Source: CAD feature listing. Evaluate the final solid. Frame: model axes, mm. A direction names the side the tool comes from. Round coordinates to 2 decimals unless told otherwise and drop trailing zeros. Write each loop counter-clockwise with the first axis right and the second up, starting at its lowest first coordinate (ties: lowest second). Pieces come first, ordered by that corner, then holes. Notation, with made-up numbers: (10.25, 33.25) -> (53.25, 33.25) arc R32 ccw to (53.25, 59.25) -> close; hole circle Ø10 at (9.25, -26.75). An arc over 180 degrees is marked (long way). Put each result on its own line as item: value.
Autodesk Inventor part; units mm, degrees
ref_plane "YZ Plane" through (0, 0, 0) normal (1, 0, 0) x (0, 1, 0)
ref_plane "XZ Plane" through (0, 0, 0) normal (0, 1, 0) x (-1, 0, 0)
ref_plane "XY Plane" through (0, 0, 0) normal (0, 0, 1) x (1, 0, 0)
sketch "Sketch1" plane through (0, 0, 0) normal (0, 0, 1) x (1, 0, 0)
  line L0 (-30, 0) -> (30, 0) construction
  line L1 (-30, -11) -> (30, -11)
  line L2 (30, 11) -> (-30, 11)
  arc A0 (-30, 11) -> (-30, -11) centre (-30, 0) ccw
  arc A1 (30, -11) -> (30, 11) centre (30, 0) ccw
  point P0 (0, 0)
  point P1 (0, 0)
  dimension "d0" = 22
  dimension "d1" = 60
extrude "Extrusion1" add sketch "Sketch1" along normal mid plane 92
sketch "Sketch2" plane through (0, 0, 46) normal (0, 0, 1) x (1, 0, 0)
  line L0 (19, 2.5) -> (31, 2.5)
  line L1 (31, 2.5) -> (31, -2.5)
  line L2 (31, -2.5) -> (19, -2.5)
  line L3 (19, -2.5) -> (19, 2.5)
  line L4 (19, 2.5) -> (31, -2.5) construction
  line L5 (31, 2.5) -> (19, -2.5) construction
  arc A0 (30, -11) -> (30, 11) centre (30, 0) ccw
  line L6 (30, 11) -> (-30, 11)
  arc A1 (-30, 11) -> (-30, -11) centre (-30, 0) ccw
  line L7 (-30, -11) -> (30, -11)
  line L8 (-29, 0) -> (-21, 0) construction
  line L9 (-29, -1.5) -> (-21, -1.5)
  line L10 (-21, 1.5) -> (-29, 1.5)
  arc A2 (-29, 1.5) -> (-29, -1.5) centre (-29, 0) ccw
  arc A3 (-21, -1.5) -> (-21, 1.5) centre (-21, 0) ccw
  point P0 (0, 0)
  point P1 (25, 0)
  point P2 (-25, 0)
  dimension "d4" = 5
  dimension "d5" = 12
  dimension "d6" = 25
  dimension "d13" = 3
  dimension "d14" = 8
  dimension "d15" = 25
extrude "Extrusion2" cut sketch "Sketch2" against normal blind 10 contours L0 L1 L2 L3 | A2 L10 A3 L9
sketch "Sketch3" plane through (-30, 11, 46) normal (0, 1, 0) x (1, 0, 0)
  circle A0 centre (30, 18.5011) radius 7.5
  point P0 (30, 46)
  dimension "d9" = 15
extrude "Extrusion3" cut sketch "Sketch3" against normal blind 1
fillet "Fillet1" radius 1 1 edges at (-7.5, 10, 27.4989)
properties part number "power-bank"
Q1. Material intervals for line 1 (X direction, y = 0.25, z = -34.5); line 2 (Y direction, x = -32.5, z = -18.5); line 3 (X direction, y = 8.5, z = 38.5), sorted ascending. Write a range as [from, to].
Ans:
line 1: x = [-41, 41]
line 2: y = [-10.71, 10.71]
line 3: x = [-36.98, 36.98]
Q2. Pin query (flat end, axial travel): pin 1 (6.5 mm diameter, centred on x = -0.5, z = 25, fed in from +Y); pin 2 (4 mm diameter, centred on x = 26, y = 0, fed in from +Z); pin 3 (6 mm diameter, centred on y = 6, z = 3, fed in from +X). Return the tip coordinate at first contact, or that it passes through.
Ans:
pin 1: stops at y = 10
pin 2: stops at z = 36
pin 3: stops at x = 40.58
Q3. Reachability of faces 1 (the flat face through (-1, 0, -46)), 2 (the flat face through (-25, -1.5, 41)) from +Z, -Z, +X, -X, +Y, -Y: full face, straight path, thin tool, end or side. Return the list, or none.
Ans:
face 1: -Z, +X, -X, +Y, -Y
face 2: +Z
Q4. Cut plane A-A on y = 0. Output: boundary loops of the cut face in (x, z), and give its area (3 significant figures).
Ans:
outline: (-41, -46) -> (41, -46) -> (41, 46) -> (31, 46) -> (31, 36) -> (19, 36) -> (19, 46) -> (-19.5, 46) -> (-19.5, 36) -> (-30.5, 36) -> (-30.5, 46) -> (-41, 46) -> close
area: 7,310 mm^2
Q5. Draft query along Y for faces 3 (the flat face through (19, 0, 41)), 4 (the flat face through (0, 10, 27)), 5 (the cylindrical face through (-41, 0, -1)). Return one class per face: +Y half, -Y half, draft (parallel to the pull), parting line (faces both ways), or undercut.
Ans:
face 3: undercut
face 4: +Y half
face 5: parting line
Q6. Cut plane B-B on z = 0. Output: boundary loops of the cut face in (x, y).
Ans:
outline: (-30, -11) -> (30, -11) arc R11 ccw to (30, 11) -> (-30, 11) arc R11 ccw to start
Q7. Cut plane C-C on y = -7. Output: boundary loops of the cut face in (x, z).
Ans:
outline: (-38.49, -46) -> (38.49, -46) -> (38.49, 46) -> (-38.49, 46) -> close
